Geometry check sheet. Reference: the model listing, model coordinates, mm. A direction names the side the tool comes from. Coordinates: 2 decimals unless noted, no trailing zeros. Write each loop counter-clockwise with the first axis right and the second up, starting at its lowest first coordinate (ties: lowest second). Pieces come first, ordered by that corner, then holes. Notation, with made-up numbers: (30.5, 50) -> (63.5, 50) arc R20 ccw to (63.5, 54) -> close; hole circle Ø11 at (36, -4.75). An arc over 180 degrees is marked (long way). Answer in a Markdown table with one row per item. Add a question column.
Q1. Section check D-D, the plane z = -69. Record the boundary of the cut face in (x, y).
Q2. Section check A-A, the plane x = 0. Record the boundary of the cut face in (y, z).
Q3. Section check B-B, the plane z = 97. Record the boundary of the cut face in (x, y).
Q4. Tool access check on faces 1 (the face through (7, -5, 2)), 2 (the face through (0.86, 0.49, 113.08)). Record the directions out of +Z, -Z, +X, -X, +Y, -Y that give a thin tool (end or side, any length) a straight path to the whole face; none if there is none.
Q5. Release check for a two-part mould opening along Z. For faces 3 (the face through (0.86, 0.49, -110.92)), 4 (the face through (0.6, 0.4, 118)), 5 (the face through (0.86, 0.49, 99.08)), 6 (the face through (-8, -5, -2)) record: pulls with the +Z half, pulls with the -Z half, needs draft (parallel to the pull), parting line crosses it, or undercut.
Q6. Section check C-C, the plane y = -2.5. Record the boundary of the cut face in (x, z), and give its area (3 significant figures).
Q7. Thickness scan on line 1 (Z direction, x = 0, y = 0.8); line 2 (X direction, y = -5, z = 45); line 3 (Y direction, x = -2.75, z = -104.5). Record the ranges inside material, lowest first.
Q8. Gauge pin test, flat ends, axial feed: P1, Ø3.5, axis at x = 1.5, z = -46, coming from the -Y side; P2, Ø3, axis at x = 4.5, y = -4.5, coming from the +Z side. Record the tip position at first contact, or that the pin passes through.
Autodesk Inventor part; units mm, degrees
ref_plane "YZ Plane" through (0, 0, 0) normal (1, 0, 0) x (0, 1, 0)
ref_plane "XZ Plane" through (0, 0, 0) normal (0, 1, 0) x (-1, 0, 0)
ref_plane "XY Plane" through (0, 0, 0) normal (0, 0, 1) x (1, 0, 0)
sketch "Esquisse4" plane through (0, 0, 0) normal (0, 1, 0) x (-1, 0, 0)
  line L0 (-8, 118) -> (8, 118)
  line L1 (8, 118) -> (8, -118)
  line L2 (8, -118) -> (-8, -118)
  line L3 (-8, -118) -> (-8, 118)
  line L4 (-8, 118) -> (8, -118) construction
  line L5 (8, 118) -> (-8, -118) construction
  point P0 (0, 0)
  dimension "d26" = 16
  dimension "d27" = 236
extrude "Plaque3" add sketch "Esquisse4" along normal blind 1
sketch "Esquisse5" plane through (7, 1, 118) normal (1, 0, 0) x (0, 1, 0)
  line L0 (0, -236) -> (0, 0)
  line L1 (0, 0) -> (-10, 0)
  line L2 (-10, 0) -> (-10, -236)
  line L3 (-10, -236) -> (0, -236)
edge flange "Bord tombé2" height 10 angle 90 thickness 1 bend radius 1 thickness toward (1, 0, 0) relief tear relief width 1 relief depth 0.5 corner gap 1 corner form 0 edges at (8, 0, 0) (-8, 0, 0) wall of the first edge with corners at (7, 1, -118) (7, 1, 118) (7, -9, 118) (7, -9, -118)
bend "Pli2"
corner "Coin2"
sketch "Esquisse6" plane through (0, 1, 0) normal (0, 1, 0) x (1, 0, 0)
  line L0 (-6, 118) -> (6, 118)
  point P0 (0, 0)
  point P1 (0, 113)
  point P2 (0, 118)
  dimension "d39" = 5
hole "Perçage2" at (0, 1, -113) direction (0, -1, 0) diameter 4.5 depth 1
sketch "Esquisse7" plane through (0, 1, 0) normal (0, 1, 0) x (1, 0, 0)
  line L0 (-6, 118) -> (6, 118)
  point P0 (0, 0)
  point P1 (0, -97)
  point P2 (0, -111)
  dimension "d50" = 215
  dimension "d51" = 14
hole "Perçage3" at (0, 1, 97) at (0, 1, 111) direction (0, -1, 0) diameter 4.5 depth 1
equation "\"d45\" = Epaisseur"
equation "\"d57\" = Epaisseur"
equation "\"d28\" = Epaisseur"
equation "\"d29\" = LargeurGrugeage"
equation "\"d30\" = ProfondeurGrugeage"
equation "\"d31\" = RestesMinimum"
equation "\"d32\" = Rayondetransition"
equation "\"d35\" = RayonPli"
equation "\"d36\" = TailleGrugeage"
equation "\"d37\" = TailleJeu"
equation "\"d38\" = TailleRayonJacobi"
equation "\"RayonPli\" = Epaisseur"
equation "\"LargeurGrugeage\" = Epaisseur"
equation "\"ProfondeurGrugeage\" = 0.5 * Epaisseur"
equation "\"TailleGrugeage\" = 4 * Epaisseur"
equation "\"RestesMinimum\" = 2 * Epaisseur"
equation "\"Rayondetransition\" = RayonPli"
equation "\"TailleRayonJacobi\" = RayonPli"
equation "\"TailleJeu\" = Epaisseur"
properties part number "support_principal"
Calculated:
| question | item | result |
|---|---|---|
| 1 | outline | (-8, -9) -> (-7, -9) -> (-7, -1) arc R1 cw to (-6, 0) -> (6, 0) arc R1 cw to (7, -1) -> (7, -9) -> (8, -9) -> (8, -1) arc R2 ccw to (6, 1) -> (-6, 1) arc R2 ccw to (-8, -1) -> close |
| 2 | outline | (0, -118) -> (1, -118) -> (1, -115.25) -> (0, -115.25) -> close; (0, -110.75) -> (1, -110.75) -> (1, 94.75) -> (0, 94.75) -> close; (0, 99.25) -> (1, 99.25) -> (1, 108.75) -> (0, 108.75) -> close; (0, 113.25) -> (1, 113.25) -> (1, 118) -> (0, 118) -> close |
| 3 | outline | (-8, -9) -> (-7, -9) -> (-7, -1) arc R1 cw to (-6, 0) -> (-2.25, 0) -> (-2.25, 1) -> (-6, 1) arc R2 ccw to (-8, -1) -> close; (2.25, 0) -> (6, 0) arc R1 cw to (7, -1) -> (7, -9) -> (8, -9) -> (8, -1) arc R2 ccw to (6, 1) -> (2.25, 1) -> close |
| 4 | face 1 | +Z, -Z, -Y |
| 4 | face 2 | +Y, -Y |
| 5 | face 3 | undercut |
| 5 | face 4 | pulls with the +Z half |
| 5 | face 5 | undercut |
| 5 | face 6 | needs draft |
| 6 | outline | (-8, -118) -> (-7, -118) -> (-7, 118) -> (-8, 118) -> close; (7, -118) -> (8, -118) -> (8, 118) -> (7, 118) -> close |
| 6 | area | 472 mm² |
| 7 | line 1 | z = -118 to -115.25, -110.75 to 94.75, 99.25 to 108.75, 113.25 to 118 |
| 7 | line 2 | x = -8 to -7, 7 to 8 |
| 7 | line 3 | y = 0 to 1 |
| 8 | P1 | stops at y = 0 |
| 8 | P2 | passes through |
